For this review, take the finished solid that the model builds, in its own axes (mm). Face numbers are marked on the shaded views. A direction names the side the tool comes from. Coordinates: 2 decimals unless noted, no trailing zeros. Loops run counter-clockwise (first coordinate to the right, second up) from the corner with the lowest first, then second, coordinate; pieces in that order, holes last.
1. Machinability: for the marked faces 1 and 2, which of the approach directions +Z, -Z, +X, -X, +Y, -Y give a long, thin tool a straight path to every point of the face, cutting with its end or side? Answer none if there is none.
2. Take a section at A-A, the plane x = 168.5. State the section outline as (y, z) points (3 decimals).
3. Take a section at B-B, the plane x = 26. State the section outline as (y, z) points, then the cut area to 3 significant figures.
4. To check wall thickness, follow probe 1 along Z at (x, y) = (143, -0.25) (3 decimals); probe 2 along Y at (x, z) = (22, -38); probe 3 along Z at (x, y) = (22, -0.4). State the ranges of each line that lie inside material, in increasing order.
5. Clearance check with flat-ended pins moving along their axes: P1, Ø7, axis at x = 145, y = 12.5, coming from the +Z side; P2, Ø3.5, axis at x = 117, z = -23.5, coming from the +Y side; P3, Ø5, axis at x = 164.5, z = -29, coming from the +Y side. State where each tip first meets the part, or that it passes through.
6. Take a section at C-C, the plane z = -18. State the section outline as (x, y) points, then the cut area to 3 significant figures.
7. Take a section at D-D, the plane y = 14.75. State the section outline as (x, z) points.
```python
from build123d import *

# Parameters (mm, degrees)
BOSS_EXTRUDE8_DEPTH = 200
SKETCH4_R           = 1.6
CUT_EXTRUDE1_DEPTH  = 2.5
CUT_EXTRUDE2_START  = -3.5
SKETCH5_R           = 1.6
CUT_EXTRUDE2_DEPTH  = 3.5
SKETCH7_R           = 1.6
CUT_EXTRUDE3_DEPTH  = 5


with BuildPart() as part:
    # Sketch6 → Boss-Extrude8 (new body)
    with BuildSketch(Plane(origin=(0, 0, 0), x_dir=(0, 0, -1), z_dir=(1, 0, 0))):
        with BuildLine():
            Line((0, 2.5), (30, 2.5))
            ThreePointArc((30, 2.5), (33.535533906, 3.964466094), (35, 7.5))
            Line((35, 7.5), (35, 21.5))
            Line((35, 21.5), (40, 21.5))
            Line((40, 21.5), (40, -3.5))
            Line((40, -3.5), (0, -3.5))
            Line((0, -3.5), (0, 2.5))
        make_face()
    extrude(amount=BOSS_EXTRUDE8_DEPTH)

    # Sketch4 → Cut-Extrude1 (cut)
    with BuildSketch(Plane(origin=(0, 0, 0), x_dir=(1, 0, 0), z_dir=(0, 1, 0))):
        with Locations(Location((22, 23.5, 0), (0, 0, 90))):
            Circle(SKETCH4_R)
        with Locations(Location((22, 6.5, 0), (0, 0, 90))):
            Circle(SKETCH4_R)
        with Locations(Location((117, 23.5, 0), (0, 0, 90))):
            Circle(SKETCH4_R)
        with Locations(Location((117, 6.5, 0), (0, 0, 90))):
            Circle(SKETCH4_R)
        with BuildLine():
            Line((139.5, 27.975), (184.5, 27.975))
            ThreePointArc((184.5, 27.975), (186.25, 26.225), (184.5, 24.475))
            Line((184.5, 24.475), (139.5, 24.475))
            ThreePointArc((139.5, 24.475), (137.75, 26.225), (139.5, 27.975))
        make_face()
        with BuildLine():
            Line((139.5, 5.525), (184.5, 5.525))
            ThreePointArc((184.5, 5.525), (186.25, 3.775), (184.5, 2.025))
            Line((184.5, 2.025), (139.5, 2.025))
            ThreePointArc((139.5, 2.025), (137.75, 3.775), (139.5, 5.525))
        make_face()
    extrude(amount=CUT_EXTRUDE1_DEPTH, mode=Mode.SUBTRACT)

    # Sketch5 → Cut-Extrude2 (cut)
    with BuildSketch(Plane(origin=(0, 0, 0), x_dir=(1, 0, 0), z_dir=(0, 1, 0)).offset(CUT_EXTRUDE2_START)):
        with Locations(Location((22, 23.5, 0), (0, 0, 90))):
            Circle(SKETCH5_R)
        with Locations(Location((22, 6.5, 0), (0, 0, 90))):
            Circle(SKETCH5_R)
        with Locations(Location((117, 23.5, 0), (0, 0, 90))):
            Circle(SKETCH5_R)
        with Locations(Location((117, 6.5, 0), (0, 0, 90))):
            Circle(SKETCH5_R)
        with BuildLine():
            Line((184.5, 23.475), (139.5, 23.475))
            ThreePointArc((139.5, 23.475), (136.75, 26.225), (139.5, 28.975))
            Line((139.5, 28.975), (184.5, 28.975))
            ThreePointArc((184.5, 28.975), (187.25, 26.225), (184.5, 23.475))
        make_face()
        with BuildLine():
            Line((184.5, 1.025), (139.5, 1.025))
            ThreePointArc((139.5, 1.025), (136.75, 3.775), (139.5, 6.525))
            Line((139.5, 6.525), (184.5, 6.525))
            ThreePointArc((184.5, 6.525), (187.25, 3.775), (184.5, 1.025))
        make_face()
    extrude(amount=CUT_EXTRUDE2_DEPTH, mode=Mode.SUBTRACT)

    # Sketch7 → Cut-Extrude3 (cut)
    with BuildSketch(Plane.XY.offset(-35)):
        with Locations((22, 10)):
            Circle(SKETCH7_R)
        with Locations((22, 18)):
            Circle(SKETCH7_R)
        with Locations((117, 10)):
            Circle(SKETCH7_R)
        with Locations((117, 18)):
            Circle(SKETCH7_R)
    extrude(amount=-CUT_EXTRUDE3_DEPTH, mode=Mode.SUBTRACT)


solid = part.part
```
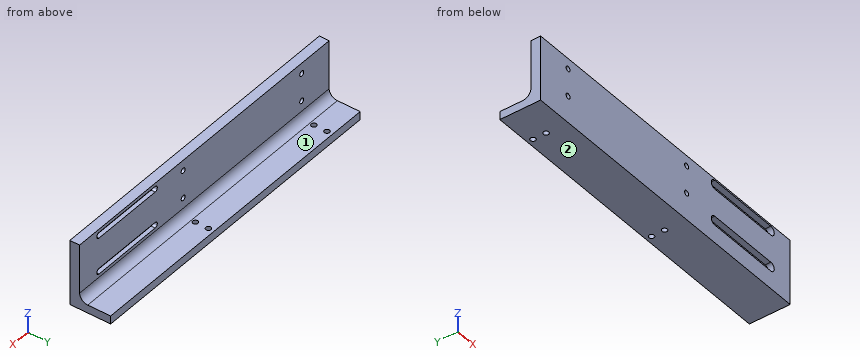
Results list:
1. face 1: +Z, +X, -X, +Y
1. face 2: -Z, +X, -X, +Y, -Y
2. outline: (-3.5, -40) - (21.5, -40) - (21.5, -35) - (7.5, -35) arc R5 cw to (2.5, -30) - (2.5, -27.975) - (0, -27.975) - (0, -28.975) - (-3.5, -28.975) - close; (-3.5, -23.475) - (0, -23.475) - (0, -24.475) - (2.5, -24.475) - (2.5, -5.525) - (0, -5.525) - (0, -6.525) - (-3.5, -6.525) - close; (-3.5, -1.025) - (0, -1.025) - (0, -2.025) - (2.5, -2.025) - (2.5, 0) - (-3.5, 0) - close
3. outline: (-3.5, -40) - (21.5, -40) - (21.5, -35) - (7.5, -35) arc R5 cw to (2.5, -30) - (2.5, 0) - (-3.5, 0) - close
3. area: 340 mm2
4. probe 1: z = -40 to -28.975, -23.475 to -6.525, -1.025 to 0
4. probe 2: y = -3.5 to 8.4, 11.6 to 16.4, 19.6 to 21.5
4. probe 3: z = -40 to -25.1, -21.9 to -8.1, -4.9 to 0
5. P1: stops at z = -35
5. P2: stops at y = 2.5
5. P3: stops at y = 2.73
6. outline: (0, -3.5) - (200, -3.5) - (200, 2.5) - (0, 2.5) - close
6. area: 1,200 mm2
7. outline: (0, -40) - (200, -40) - (200, -35) - (0, -35) - close
